For this review, take the finished solid that the model builds, in its own axes (mm). A direction names the side the tool comes from. Give positions to 0.01 mm unless a question says otherwise; leave off trailing zeros. Write each loop counter-clockwise with the first axis right and the second up, starting at its lowest first coordinate (ties: lowest second). Pieces come first, ordered by that corner, then holes.
Q1. Insertion check: P1, Ø6, axis at y = 20, z = 110.5, coming from the +X side; P2, Ø5.5, axis at x = -7.5, y = 39, coming from the +Z side; P3, Ø1.5, axis at x = -26.5, z = 82, coming from the -Y side. Each pin has a flat end and moves straight along its axis. Give the tip position at first contact, or say it passes through.
Q2. We need section A-A (x = -24). Write out the cut boundary in (y, z).
Q3. We need section D-D (z = 26). Write out the cut boundary in (x, y).
Q4. Mouldability with a two-part tool opening along Y and no side actions: class faces 1 (the flat face through (-19.5, 38, 119)), 2 (the flat face through (-1, 17, 64)), 3 (the flat face through (-18, 35, 125)) as released by +Y, released by -Y, zero draft, split by the parting line, or undercut.
Q5. Machinability: for faces 4 (the flat face through (-34, 17, 64)), 5 (the flat face through (-35.57, 37.86, 118.64)), 6 (the flat face through (0.57, 37.86, 118.64)), which of the approach directions +Z, -Z, +X, -X, +Y, -Y give a long, thin tool a straight path to every point of the face, cutting with its end or side? Answer none if there is none.
Q6. We need section B-B (x = -7.5). Give the number of separate pieces and of enclosed holes in the cut face, then the cut area to 3 significant figures.
Q7. We need section C-C (y = -4). Write out the cut boundary in (x, z), then the cut area to 3 significant figures.
Q8. For line 1 (Y direction, x = -12.5, z = 74); line 2 (X direction, y = 1.5, z = 93); line 3 (Y direction, x = -7, z = 122), list the stretches that pass through material, from the lowest coordinate up.
```python
from build123d import *

# Parameters (mm, degrees)
SKETCH_W        = 35
SKETCH_H        = 35
SKETCH_W_2      = 26
SKETCH_H_2      = 3
PAD_DEPTH       = 1.5
SKETCH001_W     = 35
SKETCH001_H     = 35
SKETCH001_W_2   = 33
SKETCH001_H_2   = 33
PAD001_DEPTH    = 120
CHAMFER_SIZE    = 1.5
SKETCH002_W     = 38
SKETCH002_H     = 50
SKETCH002_R     = 1.75
SKETCH002_W_2   = 33
SKETCH002_H_2   = 33
PAD002_DEPTH    = 2
SKETCH003_W     = 35
SKETCH003_H     = 35
SKETCH003_W_2   = 33
SKETCH003_H_2   = 33
PAD003_DEPTH    = 4
CHAMFER001_SIZE = 0.5
SKETCH004_W     = 4
SKETCH004_H     = 7.5
PAD004_DEPTH    = 7.5
CHAMFER002_SIZE = 7.4
CHAMFER003_SIZE = 1.4


with BuildPart() as part:
    # Sketch → Pad (new body)
    with BuildSketch(Plane.XY):
        with Locations((-17.5, 17.5)):
            Rectangle(SKETCH_W, SKETCH_H)
        with Locations((-17.5, 8.5)):
            Rectangle(SKETCH_W_2, SKETCH_H_2, mode=Mode.SUBTRACT)
    extrude(amount=PAD_DEPTH)

    # Sketch001 (on Face10 of Pad) → Pad001 (join)
    with BuildSketch(Plane.XY.offset(1.5)):
        with Locations((-17.5, 17.5)):
            Rectangle(SKETCH001_W, SKETCH001_H)
        with Locations((-17.5, 17.5)):
            Rectangle(SKETCH001_W_2, SKETCH001_H_2, mode=Mode.SUBTRACT)
    extrude(amount=PAD001_DEPTH)

    # Chamfer
    chamfer_edges = [part.edges().sort_by_distance(p)[0] for p in [
        (-17.5, 1, 1.5),
        (-34, 17.5, 1.5),
        (-1, 17.5, 1.5),
        (-17.5, 34, 1.5),
    ]]
    chamfer(chamfer_edges, length=CHAMFER_SIZE)

    # Sketch002 (on Face15 of Chamfer) → Pad002 (join)
    with BuildSketch(Plane.XY.offset(121.5)):
        with Locations((-17.5, 17.5)):
            Rectangle(SKETCH002_W, SKETCH002_H)
        with Locations((-27.5, -4)):
            Circle(SKETCH002_R, mode=Mode.SUBTRACT)
        with Locations((-7.5, -4)):
            Circle(SKETCH002_R, mode=Mode.SUBTRACT)
        with Locations((-27.5, 39)):
            Circle(SKETCH002_R, mode=Mode.SUBTRACT)
        with Locations((-7.5, 39)):
            Circle(SKETCH002_R, mode=Mode.SUBTRACT)
        with Locations((-17.5, 17.5)):
            Rectangle(SKETCH002_W_2, SKETCH002_H_2, mode=Mode.SUBTRACT)
    extrude(amount=PAD002_DEPTH)

    # Sketch003 (on Face17 of Pad002) → Pad003 (join)
    with BuildSketch(Plane.XY.offset(123.5)):
        with Locations((-17.5, 17.5)):
            Rectangle(SKETCH003_W, SKETCH003_H)
        with Locations((-17.5, 17.5)):
            Rectangle(SKETCH003_W_2, SKETCH003_H_2, mode=Mode.SUBTRACT)
    extrude(amount=PAD003_DEPTH)

    # Chamfer001
    chamfer001_edges = [part.edges().sort_by_distance(p)[0] for p in [
        (-35, 17.5, 127.5),
        (-17.5, 0, 127.5),
        (-17.5, 35, 127.5),
        (0, 17.5, 127.5),
    ]]
    chamfer(chamfer001_edges, length=CHAMFER001_SIZE)

    # Sketch004 (on Face32 of Chamfer001) → Pad004 (join)
    with BuildSketch(Plane(origin=(0, 0, 121.5), x_dir=(1, 0, 0), z_dir=(0, 0, -1))):
        Polygon((-35, 0), (-36.5, 7.5), (-32.5, 7.5), (-32.5, 0), align=None)
        Polygon((0, 0), (1.5, 7.5), (-2.5, 7.5), (-2.5, 0), align=None)
        with Locations((-17.5, 3.75)):
            Rectangle(SKETCH004_W, SKETCH004_H)
        Polygon((-35, -35), (-36.5, -42.5), (-32.5, -42.5), (-32.5, -35), align=None)
        Polygon((0, -35), (1.5, -42.5), (-2.5, -42.5), (-3.628958, -35), align=None)
        with Locations((-17.5, -38.75)):
            Rectangle(SKETCH004_W, SKETCH004_H)
    extrude(amount=PAD004_DEPTH)

    # Chamfer002
    chamfer002_edges = [part.edges().sort_by_distance(p)[0] for p in [
        (-34.5, -7.5, 114),
        (-17.5, -7.5, 114),
        (-0.5, -7.5, 114),
        (-34.5, 42.5, 114),
        (-17.5, 42.5, 114),
        (-0.5, 42.5, 114),
    ]]
    chamfer(chamfer002_edges, length=CHAMFER002_SIZE)

    # Chamfer003
    chamfer003_edges = [part.edges().sort_by_distance(p)[0] for p in [
        (-35, 17.5, 121.5),
        (0, 17.5, 121.5),
    ]]
    chamfer(chamfer003_edges, length=CHAMFER003_SIZE)


solid = part.part
```
Computed:
1. P1: stops at x = 0
1. P2: stops at z = 123.5
1. P3: stops at y = 0
2. outline: (-7.5, 121.5) - (0, 121.5) - (0, 0) - (7, 0) - (7, 1.5) - (2.5, 1.5) - (1, 3) - (1, 127.5) - (0.5, 127.5) - (0, 127) - (0, 123.5) - (-7.5, 123.5) - close; (10, 0) - (35, 0) - (35, 121.5) - (42.5, 121.5) - (42.5, 123.5) - (35, 123.5) - (35, 127) - (34.5, 127.5) - (34, 127.5) - (34, 3) - (32.5, 1.5) - (10, 1.5) - close
3. outline: (-35, 0) - (0, 0) - (0, 35) - (-35, 35) - close; hole (-34, 1) - (-1, 1) - (-1, 34) - (-34, 34) - close
4. face 1: zero draft
4. face 2: undercut
4. face 3: released by +Y
5. face 4: +Z
5. face 5: -Z, -X
5. face 6: -Z, +X
6. separate pieces: 4
6. enclosed holes: 0
6. area: 318 mm2
7. outline: (-36.5, 121.5) - (-36.4, 121.5) - (-35.8, 120.9) - (-35.8, 117.9) - (-32.5, 117.9) - (-32.5, 121.5) - (-29.25, 121.5) - (-29.25, 123.5) - (-36.5, 123.5) - close; (-25.75, 121.5) - (-19.5, 121.5) - (-19.5, 117.9) - (-15.5, 117.9) - (-15.5, 121.5) - (-9.25, 121.5) - (-9.25, 123.5) - (-25.75, 123.5) - close; (-5.75, 121.5) - (-2.5, 121.5) - (-2.5, 117.9) - (0.8, 117.9) - (0.8, 120.9) - (1.4, 121.5) - (1.5, 121.5) - (1.5, 123.5) - (-5.75, 123.5) - close
7. area: 101 mm2
8. line 1: y = 0 to 1, 34 to 35
8. line 2: x = -35 to -34, -1 to 0
8. line 3: y = -7.5 to -5.68, -2.32 to 1, 34 to 37.32, 40.68 to 42.5
